Geometry: final body of the model. Coordinates: model frame, mm. A direction names the side the tool comes from. Round coordinates to 2 decimals unless told otherwise and drop trailing zeros. Loops run counter-clockwise (first coordinate to the right, second up) from the corner with the lowest first, then second, coordinate; pieces in that order, holes last. Notation, with made-up numbers: (-10.75, 34.25) -> (7.25, 34.25) arc R31 cw to (7.25, 64.25) -> close; hole circle Ø9 at (22.5, 70.5). An arc over 180 degrees is marked (long way). Answer in a Markdown table with one row per item.
Autodesk Inventor part; units mm, degrees
ref_plane "YZ Plane" through (0, 0, 0) normal (1, 0, 0) x (0, 1, 0)
ref_plane "XZ Plane" through (0, 0, 0) normal (0, 1, 0) x (-1, 0, 0)
ref_plane "XY Plane" through (0, 0, 0) normal (0, 0, 1) x (1, 0, 0)
sketch "Sketch1" plane through (0, 0, 0) normal (0, 0, 1) x (1, 0, 0)
  line L0 (0, 5) -> (-5, 5)
  line L1 (-5, 5) -> (-5, 0)
  line L2 (-5, 0) -> (-25, 0)
  line L3 (-25, 0) -> (-25, -25)
  line L4 (-25, -25) -> (25, -25)
  line L5 (25, -25) -> (25, 0)
  line L6 (25, 0) -> (5, 0)
  line L7 (5, 0) -> (5, 5)
  line L8 (5, 5) -> (0, 5)
  point P0 (0, 0)
  dimension "d0" = 5
  dimension "d1" = 5
  dimension "d2" = 5
  dimension "d3" = 5
  dimension "d4" = 50
  dimension "d5" = 25
  dimension "d6" = 25
  dimension "d7" = 20
  dimension "d8" = 5
extrude "Extrusion1" add sketch "Sketch1" along normal mid plane 1000
sketch "Sketch2" plane through (25, -25, 500) normal (1, 0, 0) x (0, 0, -1)
  circle A0 centre (500, 12.5) radius 10
  line L0 (1000, 0) -> (0, 0)
  line L1 (0, 0) -> (0, 25)
  point P0 (500, 25)
  dimension "d11" = 20
  dimension "d12" = 12.5
  dimension "d13" = 500
extrude "Extrusion2" add sketch "Sketch2" along normal blind 200
properties part number "peam"
Item 1: Ray query, L1, parallel to X at y = -23.5, z = 153; L2, parallel to X at y = 1, z = 105.5; L3, parallel to Y at x = -12, z = 214.5. Return the intervals inside material, ascending.
Ans:
| item | result |
|---|---|
| L1 | -25 to 25 |
| L2 | -5 to 5 |
| L3 | -25 to 0 |
Item 2: Section query B-B, the plane y = -12.5. Output: boundary loops of the cut face in (x, z), and give its area (3 significant figures).
Ans:
| item | result |
|---|---|
| outline | (-25, -500) -> (25, -500) -> (25, -10) -> (225, -10) -> (225, 10) -> (25, 10) -> (25, 500) -> (-25, 500) -> close |
| area | 54,000 mm2 |
Item 3: Set-up query: faces 1 (the cylindrical face through (123.6, -2.74, 2.17)), 2 (the flat face through (0, -13, -500)), 3 (the flat face through (15, 0, -7)), 4 (the flat face through (-15, 0, -7)). Return all of +Z, -Z, +X, -X, +Y, -Y with unobstructed straight access to the full face (end or side cutting, diameter ignored); none if empty.
Ans:
| item | result |
|---|---|
| face 1 | +X |
| face 2 | -Z, +X, -X, +Y, -Y |
| face 3 | +Z, -Z, +X, +Y |
| face 4 | +Z, -Z, -X, +Y |
Item 4: Section query A-A, the plane z = 26. Output: boundary loops of the cut face in (x, y).
Ans:
| item | result |
|---|---|
| outline | (-25, -25) -> (25, -25) -> (25, 0) -> (5, 0) -> (5, 5) -> (-5, 5) -> (-5, 0) -> (-25, 0) -> close |
Item 5: Section query C-C, the plane x = 149. Output: boundary loops of the cut face in (y, z).
Ans:
| item | result |
|---|---|
| outline | circle Ø20 at (-12.5, 0) |
Item 6: First-contact query: P1, Ø10, axis at x = -18, z = 26.5, coming from the +Y side; P2, Ø4, axis at y = -3.5, z = 380.5, coming from the +X side; P3, Ø6, axis at x = 116, y = -19, coming from the +Z side. Flat tips, straight axial feed; report the tip coordinate or a pass-through.
Ans:
| item | result |
|---|---|
| P1 | y = 0 |
| P2 | x = 25 |
| P3 | z = 9.37 |
